from build123d import *

# Parameters (mm, degrees)
EXTRUDE1_DEPTH          = 17.5
SKETCH2_W               = 75
SKETCH2_H               = 15
CUT_EXTRUDE1_DEPTH      = 330.289006801
CUT_EXTRUDE2_DEPTH      = 327.429548295
CUT_EXTRUDE2_DEPTH_BACK = 327.429548295
SKETCH3_R               = 5
CUT_EXTRUDE3_DEPTH      = 327.429548295
CUT_EXTRUDE3_DEPTH_BACK = 327.429548295
SKETCH4_W               = 255
SKETCH4_H               = 30


with BuildPart() as part:
    # Sketch1 → Extrude1 (new, symmetric)
    with BuildSketch(Plane.XY):
        with BuildLine():
            Line((-10, 25), (325, 25))
            Line((325, 25), (325, -25))
            Line((325, -25), (-10, -25))
            ThreePointArc((-10, -25), (-20.606601718, -20.606601718), (-25, -10))
            Line((-25, -10), (-25, 10))
            ThreePointArc((-25, 10), (-20.606601718, 20.606601718), (-10, 25))
        make_face()
    extrude(amount=EXTRUDE1_DEPTH, both=True)

    # Sketch2 → Cut-Extrude1 (cut, through all)
    with BuildSketch(Plane(origin=(0, 25, 0), x_dir=(-1, 0, 0), z_dir=(0, 1, 0))):
        with Locations((-12.5, 0)):
            Rectangle(SKETCH2_W, SKETCH2_H)
    extrude(amount=-CUT_EXTRUDE1_DEPTH, mode=Mode.SUBTRACT)

    # Sketch3 → Cut-Extrude2 (cut, two sides: drawn at the far end of the back side and taken through both)
    with BuildSketch(Plane.XY.offset(-CUT_EXTRUDE2_DEPTH_BACK)):
        Circle(SKETCH3_R)
    extrude(amount=CUT_EXTRUDE2_DEPTH + CUT_EXTRUDE2_DEPTH_BACK, mode=Mode.SUBTRACT)

    # Sketch4 → Cut-Extrude3 (cut, two sides: drawn at the far end of the back side and taken through both)
    with BuildSketch(Plane.XY.offset(-CUT_EXTRUDE3_DEPTH_BACK)):
        with Locations((187.5, 0)):
            Rectangle(SKETCH4_W, SKETCH4_H)
    extrude(amount=CUT_EXTRUDE3_DEPTH + CUT_EXTRUDE3_DEPTH_BACK, mode=Mode.SUBTRACT)


solid = part.part
Part model, mm, in its own coordinate system. A direction names the side the tool comes from. Give positions to 0.01 mm unless a question says otherwise; leave off trailing zeros. Order: outer loops, then holes, each group sorted by start corner. A loop starts at its lowest first (then second) coordinate and runs counter-clockwise, first axis right, second up. Notation, with made-up numbers: (71.5, -12) - (93.5, -12) arc R13 cw to (93.5, -2) - close; hole circle Ø2 at (48, 68.5). An arc over 180 degrees is marked (long way). One line per question, with ' | ' between items.
1. Band-saw the part on B-B on z = 0. List the corners of the cut face in (x, y).
Filled in:
outline: (50, -25) - (325, -25) - (325, 25) - (50, 25) - close; hole (60, -15) - (315, -15) - (315, 15) - (60, 15) - close
2. Drop flat-ended pins along their axis: P1, Ø10, axis at x = 72.5, y = 6.5, coming from the +Z side; P2, Ø4, axis at y = -3.5, z = 3, coming from the -X side. Give the stop position or say it passes through.
Filled in:
P1: through | P2: x = 50
3. Band-saw the part on C-C on y = 0. List the corners of the cut face in (x, z), then the cut area to 3 significant figures.
Filled in:
outline: (-25, -17.5) - (-5, -17.5) - (-5, -7.5) - (-25, -7.5) - close; (-25, 7.5) - (-5, 7.5) - (-5, 17.5) - (-25, 17.5) - close; (5, -17.5) - (60, -17.5) - (60, 17.5) - (5, 17.5) - (5, 7.5) - (50, 7.5) - (50, -7.5) - (5, -7.5) - close; (315, -17.5) - (325, -17.5) - (325, 17.5) - (315, 17.5) - close | area: 2,000 mm²
4. Pull direction X, two halves, no side cores. Call faces 1 (the face through (-25, 0, 13)), 2 (the face through (13, 0, -7.5)), 3 (the face through (-1.08, -4.88, 12.43)): +X half, -X half, draft (parallel to the pull), parting line (faces both ways), or undercut.
Filled in:
face 1: -X half | face 2: draft | face 3: undercut
5. Drill centre lines: probe 1 along X at (y, z) = (0, -9.75); probe 2 along Y at (x, z) = (0, -11); probe 3 along X at (y, z) = (-7, 1). Where is each one in solid material? Low to high.
Filled in:
probe 1: -25 to -5, 5 to 60, 315 to 325 | probe 2: -25 to -5, 5 to 25 | probe 3: 50 to 60, 315 to 325
6. Band-saw the part on D-D on x = 186. List the corners of the cut face in (y, z), then the cut area to 3 significant figures.
Filled in:
outline: (-25, -17.5) - (-15, -17.5) - (-15, 17.5) - (-25, 17.5) - close; (15, -17.5) - (25, -17.5) - (25, 17.5) - (15, 17.5) - close | area: 700 mm²
7. Band-saw the part on A-A on x = 0. List the corners of the cut face in (y, z), then the cut area to 3 significant figures.
Filled in:
outline: (-25, -17.5) - (-5, -17.5) - (-5, -7.5) - (-25, -7.5) - close; (-25, 7.5) - (-5, 7.5) - (-5, 17.5) - (-25, 17.5) - close; (5, -17.5) - (25, -17.5) - (25, -7.5) - (5, -7.5) - close; (5, 7.5) - (25, 7.5) - (25, 17.5) - (5, 17.5) - close | area: 800 mm²
8. Which spindle directions (+Z, -Z, +X, -X, +Y, -Y) get a long thin tool onto all of the face, cutting with end or side? Do faces 4 (the face through (13, 0, 7.5)), 5 (the face through (114, 17, 17.5)), 6 (the face through (186, 15, 0)). Say none if no direction does.
Filled in:
face 4: -X, +Y, -Y | face 5: +Z, +X, -X, +Y, -Y | face 6: +Z, -Z
